```python
from build123d import *

# Parameters (mm, degrees)
SKETCH1_R           = 2.286
BOSS_EXTRUDE1_DEPTH = 76.2
SKETCH2_W           = 19.05
SKETCH2_H           = 63.5
SKETCH2_H_2         = 6.35
CUT_EXTRUDE1_DEPTH  = 102.60793719
SKETCH3_W           = 25.4
SKETCH3_H           = 6.858
CUT_EXTRUDE2_DEPTH  = 100.367382835
FILLET1_R           = 1.27
FILLET2_R           = 12.7
SKETCH4_W           = 59.009552573
SKETCH4_H           = 74.343024825
CUT_EXTRUDE3_DEPTH  = 85.041380514


with BuildPart() as part:
    # Sketch1 → Boss-Extrude1 (new body)
    with BuildSketch(Plane(origin=(0, 0, 0), x_dir=(1, 0, 0), z_dir=(0, 1, 0))):
        with BuildLine():
            Line((-5.679612663, -2.839806331), (-24.729612663, 35.260193669))
            ThreePointArc((-24.729612663, 35.260193669), (-25.238895582, 39.521292183), (-22.921549668, 43.133249763))
            Line((-22.921549668, 43.133249763), (-6.35, 55.88))
            Line((-6.35, 55.88), (12.7, 55.88))
            ThreePointArc((12.7, 55.88), (18.555327731, 55.700289554), (24.388613689, 55.161834718))
            ThreePointArc((24.388613689, 55.161834718), (8.638623245, 35.753941369), (12.7, 11.091546065))
            Line((12.7, 11.091546065), (5.670682494, -2.857596902))
            ThreePointArc((5.670682494, -2.857596902), (-0.009953044, -6.3499922), (-5.679612663, -2.839806331))
        make_face()
        with Locations(Location((0, 0, 0), (0, 0, 90))):
            Circle(SKETCH1_R, mode=Mode.SUBTRACT)
        with Locations(Location((-19.05, 38.1, 0), (0, 0, 90))):
            Circle(SKETCH1_R, mode=Mode.SUBTRACT)
    extrude(amount=BOSS_EXTRUDE1_DEPTH)

    # Sketch2 → Cut-Extrude1 (cut, through all)
    with BuildSketch(Plane(origin=(0, 0, -55.88), x_dir=(-1, 0, 0), z_dir=(0, 0, -1))):
        with Locations((15.875, 31.75)):
            Rectangle(SKETCH2_W, SKETCH2_H)
        with Locations((15.875, 73.025)):
            Rectangle(SKETCH2_W, SKETCH2_H_2)
    extrude(amount=-CUT_EXTRUDE1_DEPTH, mode=Mode.SUBTRACT)

    # Sketch3 → Cut-Extrude2 (cut, through all)
    with BuildSketch(Plane.ZY.offset(6.35)):
        with Locations((-6.35, 53.975)):
            Rectangle(SKETCH3_W, SKETCH3_H)
    extrude(amount=-CUT_EXTRUDE2_DEPTH, mode=Mode.SUBTRACT)

    # Fillet1
    fillet1_edges = [part.edges().sort_by_distance(p)[0] for p in [
        (24.388613689, 38.1, -55.161834718),
    ]]
    fillet(fillet1_edges, radius=FILLET1_R)

    # Fillet2
    fillet2_edges = [part.edges().sort_by_distance(p)[0] for p in [
        (12.7, 66.802, -11.091546065),
        (12.7, 25.273, -11.091546065),
    ]]
    fillet(fillet2_edges, radius=FILLET2_R)

    # Sketch4 → Cut-Extrude3 (cut, through all)
    with BuildSketch(Plane.XZ.offset(-57.404)):
        with Locations((-1.749174137, -25.683599477)):
            Rectangle(SKETCH4_W, SKETCH4_H)
    extrude(amount=CUT_EXTRUDE3_DEPTH, mode=Mode.SUBTRACT)


solid = part.part
```
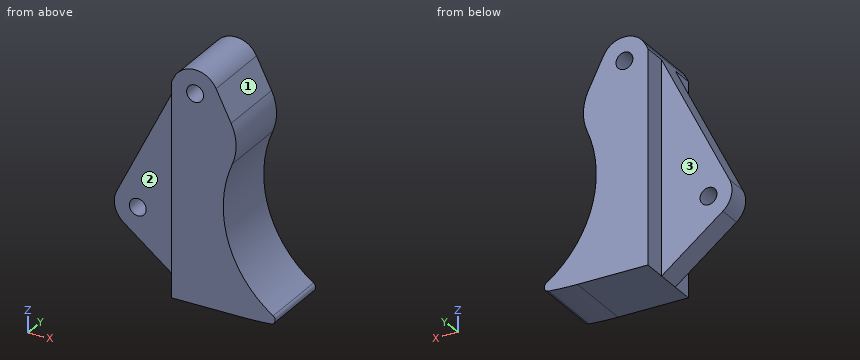
Build history of the part. All positions in model axes, mm. Face numbers are marked on the shaded views. A direction names the side the tool comes from. Coordinates: 2 decimals unless noted, no trailing zeros. Order: outer loops, then holes, each group sorted by start corner. A loop starts at its lowest first (then second) coordinate and runs counter-clockwise, first axis right, second up. Notation, with made-up numbers: M 17,34.5 L 49,34.5 A32 cw 49,64.5 Z; hole C 0,-27.5 d1. An arc over 180 degrees is marked long. One line per question, with ' | ' between items. Start each with the question number.
1. Cut at D-D (z = -18.5). Write the cut outline in (x, y), plus the area to 3 significant figures.
2. Cut at A-A (x = -19.05). Write the cut outline in (y, z).
3. Tool access for the marked faces 1, 2 and 3: list every direction of +Z, -Z, +X, -X, +Y, -Y with a clear straight run to the whole face (end or side of a thin tool).
4. Cut at C-C (x = 0). Write the cut outline in (y, z), plus the area to 3 significant figures.
5. Flat gauge pins, fed straight in: P1, Ø1.5, axis at x = -20, z = -25, coming from the +Y side; P2, Ø7, axis at y = 72.5, z = -27, coming from the -X side; P3, Ø3, axis at x = -20, y = 73, coming from the +Z side; P4, Ø12, axis at x = -15.5, z = -24, coming from the -Y side. Where does each tip first touch, or does it go through?
6. Wall check: line 1 along Y through (x, z) = (-14.5, -39.5); line 2 along X through (y, z) = (72.5, 2); line 3 along X through (y, z) = (65.5, -38.1). Give the ranges that are in metal, low to high. Write a range as [from, to].
7. Cut at B-B (z = -38.1). Write the cut outline in (x, y).
The answers:
1) outline: M -16.35,63.5 L -6.35,63.5 L -6.35,57.4 L 9.12,57.4 L 9.12,76.2 L -6.35,76.2 L -6.35,69.85 L -16.35,69.85 Z | area: 354 mm2
2) outline: M 63.5,-46.11 L 69.85,-46.11 L 69.85,-40.39 L 63.5,-40.39 Z; M 63.5,-35.81 L 69.85,-35.81 L 69.85,-23.9 L 63.5,-23.9 Z
3) face 1: +Z, +X, +Y, -Y | face 2: +Z, -Z, -X, -Y | face 3: +Z, -Z, -X, +Y
4) outline: M 57.4,-55.88 L 76.2,-55.88 L 76.2,-2.29 L 57.4,-2.29 Z; M 57.4,2.29 L 76.2,2.29 L 76.2,6.35 L 57.4,6.35 Z | area: 1,080 mm2
5) P1: stops at y = 69.85 | P2: stops at x = -21.74 | P3: passes through | P4: stops at y = 63.5
6) line 1: y = [63.5, 69.85] | line 2: x = [-6.1, -1.11], [1.11, 6.1] | line 3: x = [-25.4, -21.34], [-16.76, 9.36]
7) outline: M -25.4,63.5 L -21.34,63.5 L -21.34,69.85 L -25.4,69.85 Z; M -16.76,63.5 L -6.35,63.5 L -6.35,57.4 L 9.36,57.4 L 9.36,76.2 L -6.35,76.2 L -6.35,69.85 L -16.76,69.85 Z
